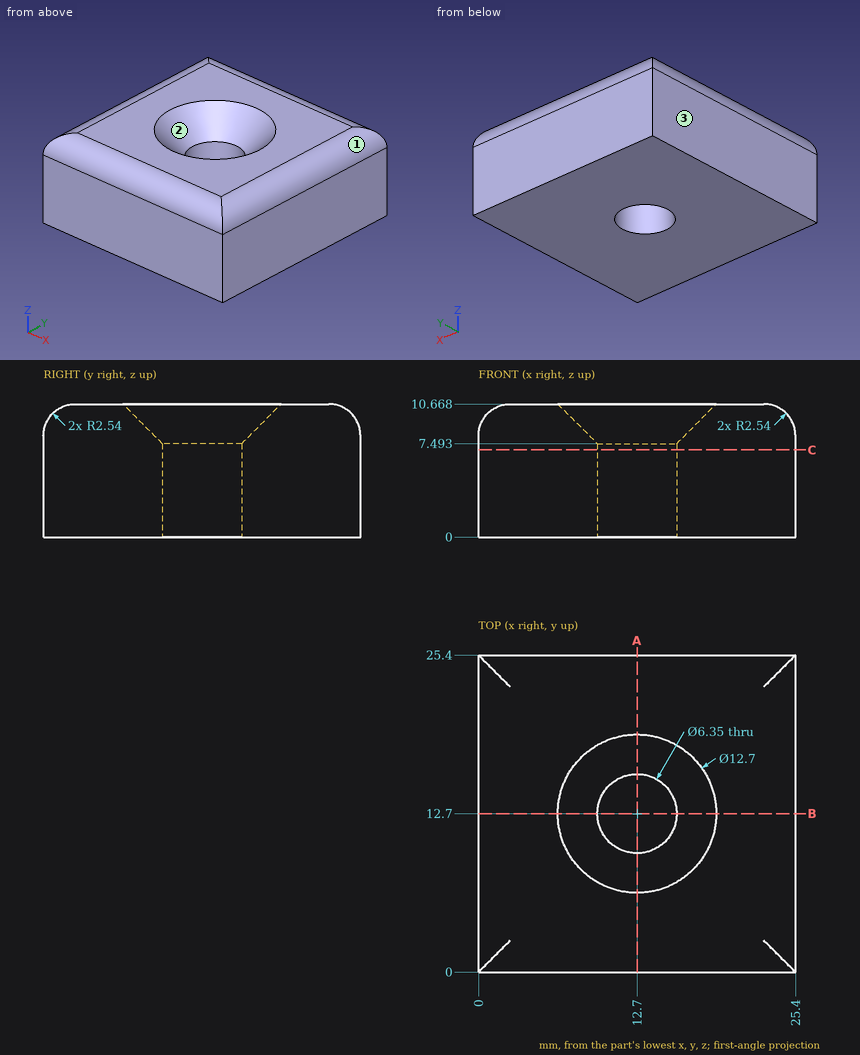
Could you check a few things on this drawing? It's one solid part, dimensions in mm from its lowest x, y, z. Round coordinates to 2 decimals unless told otherwise and drop trailing zeros. Write each loop counter-clockwise with the first axis right and the second up, starting at its lowest first coordinate (ties: lowest second). Pieces come first, ordered by that corner, then holes. Notation, with made-up numbers: (8, -29) -> (27, -29) arc R15 ccw to (27, -9) -> close; hole circle Ø3 at (58.5, 86). An arc over 180 degrees is marked (long way). Use one line per item in the form item = value. Start each with the question number.
Q1. Imagine slicing it at A-A (x = 12.7). Please give me the cut outline in (y, z) (3 decimals).
Q2. We'd pull the mould along X, two halves only. Please class the marked faces 1, 2 and 3: +X half, -X half, draft (parallel to the pull), parting line (faces both ways), or undercut.
Q3. If I drill on probe 1 along X at (y, z) = (12.7, 3.5) (3 decimals); probe 2 along Y at (x, z) = (14.5, 2.5), over which ranges is the centre line in solid material (lowest first)? Write a range as [from, to].
Q4. Imagine slicing it at C-C (z = 7). Please give me the cut outline in (x, y) (3 decimals), then the cut area to 3 significant figures.
Worked out:
q1.outline = (0, 0) -> (9.525, 0) -> (9.525, 7.493) -> (6.35, 10.668) -> (2.54, 10.668) arc R2.54 ccw to (0, 8.128) -> close; (15.875, 0) -> (25.4, 0) -> (25.4, 8.128) arc R2.54 ccw to (22.86, 10.668) -> (19.05, 10.668) -> (15.875, 7.493) -> close
q2.face_1 = +X half
q2.face_2 = undercut
q2.face_3 = -X half
q3.probe_1 = [0, 9.525], [15.875, 25.4]
q3.probe_2 = [0, 10.08], [15.32, 25.4]
q4.outline = (0, 0) -> (25.4, 0) -> (25.4, 25.4) -> (0, 25.4) -> close; hole circle Ø6.35 at (12.7, 12.7)
q4.area = 613 mm^2
